The listing builds one solid part. Answer for the finished solid, in the listing's coordinates (mm). A direction names the side the tool comes from. Give positions to 0.01 mm unless a question says otherwise; leave off trailing zeros. Loops run counter-clockwise (first coordinate to the right, second up) from the corner with the lowest first, then second, coordinate; pieces in that order, holes last. Notation, with made-up numbers: M 49,2.25 L 77,2.25 A9 cw 77,11.25 Z; hole C -4,63.25 d4. An arc over 180 degrees is marked long. Use one line per item in the form item = value. Start each with the question number.
1. For faces 1 (the face through (-2.5, 0.644, 2.4)), 2 (the face through (2.757, 3.197, 1.759)), 3 (the face through (-2.5, 0.644, -2.4)), determine the directions among +Z, -Z, +X, -X, +Y, -Y from which every point of the face is accessible in a straight line to the end or side of a thin tool.
2. Each of these flat-tipped pins is pushed along its axis until it touches: pin 1 Ø2 at (x, z) = (1.5, 0.5) entering from -Y; pin 2 Ø2.5 at (x, z) = (-2, 2.5) entering from +Y; pin 3 Ø1 at (x, z) = (2.5, -2.5) entering from +Y; pin 4 Ø2 at (x, y) = (1.5, 4) entering from -Z. Where does it stop, or does it pass through?
3. The part is cut by section D-D (y = 4.7). Write down the section's boundary in (x, z), and give its area (3 significant figures).
4. Straight lines are drawn through the part: line 1 (Y direction, x = -3, z = 2.5); line 2 (Y direction, x = 0.5, z = -1.25); line 3 (Z direction, x = 1.25, y = 4.8). For each, find the intervals that lie inside material, in ascending order. Write a range as from..to.
5. The part is cut by section B-B (y = 0.2). Write down the section's boundary in (x, z) (3 decimals), and give its area (3 significant figures).
from build123d import *

# Parameters (mm, degrees)
BOSS_EXTRUDE1_DEPTH = 0.1571
BOSS_EXTRUDE2_DEPTH = 0.6443
CHAMFER1_SIZE       = 0.0487
BOSS_EXTRUDE3_START = -0.1571
BOSS_EXTRUDE3_DEPTH = 0.0514
SKETCH2_R           = 3.27
BOSS_EXTRUDE4_DEPTH = 5.5
CHAMFER2_SIZE       = 0.2155
CHAMFER2_SIZE2      = 0.314


with BuildPart() as part:
    # Sketch1 → Boss-Extrude1 (new body)
    with BuildSketch(Plane(origin=(0, 0, 0), x_dir=(1, 0, 0), z_dir=(0, 1, 0))):
        Polygon((-1.115015984, 1.105000019), (-1.120023966, 3.314999898), (-2.051918983, 3.314999898), (-3.314999898, 2.002368291), (-3.314999898, 1.098344008), align=None)
        Polygon((0, -1.592377345), (0, 1.592377345), (-0.288244069, 1.592377345), (-0.28754435, 3.314999898), (-1.120023966, 3.314999898), (-1.115015984, 1.105000019), (-3.314999898, 1.098344008), (-3.314999898, -1.118712743), (-1.110008001, -1.105000019), (-1.105000019, -3.314999898), (-0.289643526, -3.314999898), (-0.288943807, -1.592377345), align=None)
        Polygon((-3.314999898, -3.314999898), (-1.105000019, -3.314999898), (-1.110008001, -1.105000019), (-3.314999898, -1.118712743), align=None)
        Polygon((0.288943807, -1.592377345), (0, -1.592377345), (0, -3.314999898), (0.289643526, -3.314999898), align=None)
        Polygon((0, -3.314999898), (0, -1.592377345), (-0.288943807, -1.592377345), (-0.289643526, -3.314999898), align=None)
        Polygon((0, 1.592377345), (0, 3.314999898), (-0.28754435, 3.314999898), (-0.288244069, 1.592377345), align=None)
        Polygon((0.28754435, 3.314999898), (0, 3.314999898), (0, 1.592377345), (0.288244069, 1.592377345), align=None)
        Polygon((0.288244069, 1.592377345), (0, 1.592377345), (0, -1.592377345), (0.288943807, -1.592377345), (0.289643526, -3.314999898), (1.105000019, -3.314999898), (1.110008001, -1.10500002), (3.314999898, -1.118712743), (3.314999898, 1.098344008), (1.115015984, 1.105000019), (1.120023966, 3.314999898), (0.28754435, 3.314999898), align=None)
        Polygon((2.051671346, 3.314999898), (1.120023966, 3.314999898), (1.115015984, 1.105000019), (3.314999898, 1.098344008), (3.314999898, 2.002368291), align=None)
        Polygon((1.110008001, -1.10500002), (1.105000019, -3.314999898), (3.314999898, -3.314999898), (3.314999898, -1.118712743), align=None)
    extrude(amount=-BOSS_EXTRUDE1_DEPTH)

    # Sketch1<4> → Boss-Extrude2 (add)
    with BuildSketch(Plane(origin=(0, 0, 0), x_dir=(1, 0, 0), z_dir=(0, 1, 0))):
        Polygon((-1.115015984, 1.105000019), (-1.120023966, 3.314999898), (-2.051918983, 3.314999898), (-3.314999898, 2.002368291), (-3.314999898, 1.098344008), align=None)
        Polygon((-3.314999898, -3.314999898), (-1.105000019, -3.314999898), (-1.110008001, -1.105000019), (-3.314999898, -1.118712743), align=None)
        Polygon((1.115015984, 1.105000019), (3.314999898, 1.098344008), (3.314999898, 2.002368291), (2.051671346, 3.314999898), (1.120023966, 3.314999898), align=None)
        Polygon((1.105000019, -3.314999898), (3.314999898, -3.314999898), (3.314999898, -1.118712743), (1.110008001, -1.10500002), align=None)
    extrude(amount=BOSS_EXTRUDE2_DEPTH)

    # Chamfer1
    chamfer1_edges = [part.edges().sort_by_distance(p)[0] for p in [
        (2.212503949, 0.6443, 1.111856381),
        (3.314999898, 0.6443, 2.216856321),
        (2.209999959, 0.6443, 3.314999898),
        (1.10750401, 0.6443, 2.209999959),
        (1.117519975, 0.6443, -2.209999959),
        (1.585847656, 0.6443, -3.314999898),
        (2.683335622, 0.6443, -2.658684095),
        (3.314999898, 0.6443, -1.55035615),
        (2.215007941, 0.6443, -1.101672014),
        (-2.215007941, 0.6443, -1.101672014),
        (-3.314999898, 0.6443, -1.55035615),
        (-2.683459441, 0.6443, -2.658684095),
        (-1.585971475, 0.6443, -3.314999898),
        (-1.117519975, 0.6443, -2.209999959),
        (-2.209999959, 0.6443, 3.314999898),
        (-3.314999898, 0.6443, 2.216856321),
        (-2.21250395, 0.6443, 1.111856381),
        (-1.10750401, 0.6443, 2.209999959),
    ]]
    chamfer(chamfer1_edges, length=CHAMFER1_SIZE)

    # Sketch1<5> → Boss-Extrude3 (add)
    with BuildSketch(Plane(origin=(0, 0, 0), x_dir=(1, 0, 0), z_dir=(0, 1, 0)).offset(BOSS_EXTRUDE3_START)):
        Polygon((0, -3.314999898), (0, -1.592377345), (-0.288943807, -1.592377345), (-0.289643526, -3.314999898), align=None)
        Polygon((0.288943807, -1.592377345), (0, -1.592377345), (0, -3.314999898), (0.289643526, -3.314999898), align=None)
        Polygon((0, 1.592377345), (0, 3.314999898), (-0.28754435, 3.314999898), (-0.288244069, 1.592377345), align=None)
        Polygon((0.28754435, 3.314999898), (0, 3.314999898), (0, 1.592377345), (0.288244069, 1.592377345), align=None)
    extrude(amount=-BOSS_EXTRUDE3_DEPTH)

    # Sketch2 → Boss-Extrude4 (add)
    with BuildSketch(Plane(origin=(0, 0, 0), x_dir=(1, 0, 0), z_dir=(0, 1, 0))):
        with Locations(Location((0, 0, 0), (0, 0, 69.980077841))):
            Circle(SKETCH2_R)
    extrude(amount=BOSS_EXTRUDE4_DEPTH)

    # Chamfer2
    chamfer2_edges = [part.edges().sort_by_distance(p)[0] for p in [
        (-1.119474234, 5.5, 3.072405806),
    ]]
    chamfer2_side = [part.faces().sort_by_distance(p)[0] for p in [
        (-1.119474234, 2.75, 3.072405806),
    ]]
    chamfer(chamfer2_edges, length=CHAMFER2_SIZE, length2=CHAMFER2_SIZE2, reference=chamfer2_side[0])

    # Sketch3 → Cut-Revolve1 (revolve, cut)
    with BuildSketch(Plane.XY, mode=Mode.PRIVATE) as cut_revolve1_sk:
        Polygon((3.1392, 1.0429), (3.1392, 0.9251), (3.27, 0.8), (3.27, 1.168), align=None)
    revolve(cut_revolve1_sk.sketch.rotate(Axis((0, 5.2845, 0), (0, -1, 0)), 290.019922159), axis=Axis((0, 5.2845, 0), (0, -1, 0)), mode=Mode.SUBTRACT)


solid = part.part
Derived:
q1.face_1 = +Z, -X, +Y
q1.face_2 = +Y
q1.face_3 = -Z, -X, +Y
q2.pin_1 = -0.16
q2.pin_2 = 5.5
q2.pin_3 = 5.45
q2.pin_4 = -3.23
q3.outline = C 0,0 d6.54
q3.area = 33.6 mm2
q4.line_1 = -0.16..0.64
q4.line_2 = -0.16..5.5
q4.line_3 = -3.02..3.02
q5.outline = M -3.315,-2.002 L -2.052,-3.315 L -1.12,-3.315 L -1.119,-3.072 A3.27 ccw 1.119,-3.072 L 1.12,-3.315 L 2.052,-3.315 L 3.315,-2.002 L 3.315,-1.098 L 3.08,-1.099 A3.27 ccw 3.073,1.117 L 3.315,1.119 L 3.315,3.315 L 1.105,3.315 L 1.106,3.077 A3.27 ccw -1.106,3.077 L -1.105,3.315 L -3.315,3.315 L -3.315,1.119 L -3.073,1.117 A3.27 ccw -3.08,-1.099 L -3.315,-1.098 Z
q5.area = 41.3 mm2
